from build123d import *

# Parameters (mm, degrees)
EXTRUDE_1_DEPTH     = 9
SKETCH_2_W          = 12.1
SKETCH_2_H          = 5
CUT_EXTRUDE_1_DEPTH = 0.9
SKETCH_3_R          = 29.401854515
SKETCH_3_W          = 23
SKETCH_3_H          = 15
CUT_EXTRUDE_2_DEPTH = 1
CHAMFER_1_SIZE      = 2
CUT_EXTRUDE_4_DEPTH = 7.8
SKETCH_5_W          = 12.1
SKETCH_5_H          = 1.6
CUT_EXTRUDE_5_DEPTH = 5
SKETCH_6_R          = 1
SKETCH_6_R_2        = 0.9
CUT_EXTRUDE_6_DEPTH = 3
CUT_EXTRUDE_7_DEPTH = 3
EXTRUDE_2_DEPTH     = 3
CUT_EXTRUDE_9_DEPTH = 1.7
FILLET_1_R          = 1


with BuildPart() as part:
    # Эскиз1 → Бобышка-Вытянуть1 (new body)
    with BuildSketch(Plane(origin=(0, 0, 0), x_dir=(1, 0, 0), z_dir=(0, 1, 0))):
        with BuildLine():
            Line((-13.5, 35.6), (13.5, 35.6))
            Line((13.5, 35.6), (13.5, -23.6))
            ThreePointArc((13.5, -23.6), (9.985281374, -32.085281374), (1.5, -35.6))
            Line((1.5, -35.6), (-10.5, -35.6))
            ThreePointArc((-10.5, -35.6), (-12.621320344, -34.721320344), (-13.5, -32.6))
            Line((-13.5, -32.6), (-13.5, 35.6))
        make_face()
    extrude(amount=EXTRUDE_1_DEPTH)

    # Эскиз2 → Вырез-Вытянуть1 (cut)
    with BuildSketch(Plane(origin=(0, 0, -35.6), x_dir=(-1, 0, 0), z_dir=(0, 0, -1))):
        Polygon((7.05, 6), (7.05, 0), (13.5, 0), (13.5, 9), (-13.5, 9), (-13.5, 0), (-7.05, 0), (-7.05, 6), align=None)
        with Locations((0, 2.5)):
            Rectangle(SKETCH_2_W, SKETCH_2_H)
    extrude(amount=-CUT_EXTRUDE_1_DEPTH, mode=Mode.SUBTRACT)

    # Эскиз3 → Вырез-Вытянуть2 (cut)
    with BuildSketch(Plane(origin=(0, 0, -34.7), x_dir=(-1, 0, 0), z_dir=(0, 0, -1))):
        Circle(SKETCH_3_R)
        Rectangle(SKETCH_3_W, SKETCH_3_H, mode=Mode.SUBTRACT)
    extrude(amount=-CUT_EXTRUDE_2_DEPTH, mode=Mode.SUBTRACT)

    # Фаска1
    chamfer_1_edges = [part.edges().sort_by_distance(p)[0] for p in [
        (-4.5, 9, 35.6),
        (9.985281374, 9, 32.085281374),
        (13.5, 9, -5.05),
        (-13.5, 9, -0.55),
        (-12.621320344, 9, 34.721320344),
    ]]
    chamfer(chamfer_1_edges, length=CHAMFER_1_SIZE)

    # Эскиз4 → Вырез-Вытянуть4 (cut)
    with BuildSketch(Plane.XZ):
        with BuildLine():
            Line((9.9, -33.1), (9.9, -32.1))
            Line((9.9, -32.1), (11.9, -32.1))
            Line((11.9, -32.1), (11.9, 23.6))
            ThreePointArc((11.9, 23.6), (8.853910524, 30.953910524), (1.5, 34))
            Line((1.5, 34), (-10.5, 34))
            ThreePointArc((-10.5, 34), (-11.489949494, 33.589949494), (-11.9, 32.6))
            Line((-11.9, 32.6), (-11.9, -32.1))
            Line((-11.9, -32.1), (-9.9, -32.1))
            Line((-9.9, -32.1), (-9.9, -33.1))
            Line((-9.9, -33.1), (9.9, -33.1))
        make_face()
    extrude(amount=-CUT_EXTRUDE_4_DEPTH, mode=Mode.SUBTRACT)

    # Эскиз5 → Вырез-Вытянуть5 (cut)
    with BuildSketch(Plane.XZ):
        with Locations((0, -33.9)):
            Rectangle(SKETCH_5_W, SKETCH_5_H)
    extrude(amount=-CUT_EXTRUDE_5_DEPTH, mode=Mode.SUBTRACT)

    # Эскиз6 → Вырез-Вытянуть6 (cut)
    with BuildSketch(Plane(origin=(0, 9, 0), x_dir=(1, 0, 0), z_dir=(0, 1, 0))):
        with Locations(Location((-6.5, -27.6, 0), (0, 0, 270))):
            Circle(SKETCH_6_R)
        with Locations(Location((1.5, -23.6, 0), (0, 0, 270))):
            Circle(SKETCH_6_R_2)
    extrude(amount=-CUT_EXTRUDE_6_DEPTH, mode=Mode.SUBTRACT)

    # Эскиз8 → Вырез-Вытянуть7 (cut)
    with BuildSketch(Plane(origin=(13.5, 0, 0), x_dir=(0, 0, -1), z_dir=(1, 0, 0))):
        with BuildLine():
            Line((-22.65, 2.2), (-22.65, 0))
            Line((-22.65, 0), (-18.15, 0))
            Line((-18.15, 0), (-18.15, 2.2))
            ThreePointArc((-18.15, 2.2), (-20.4, 4.45), (-22.65, 2.2))
        make_face()
    extrude(amount=-CUT_EXTRUDE_7_DEPTH, mode=Mode.SUBTRACT)

    # Эскиз10 → Бобышка-Вытянуть2 (add)
    with BuildSketch(Plane(origin=(0, 9, 0), x_dir=(1, 0, 0), z_dir=(0, 1, 0))):
        with BuildLine():
            Line((-11.5, 33.7), (11.5, 33.7))
            Line((11.5, 33.7), (4.619956712, 26.186537456))
            ThreePointArc((4.619956712, 26.186537456), (0, 24.3), (-4.619956712, 26.186537456))
            Line((-4.619956712, 26.186537456), (-11.5, 33.7))
        make_face()
    extrude(amount=-EXTRUDE_2_DEPTH)

    # Эскиз9 → Вырез-Вытянуть9 (cut)
    with BuildSketch(Plane(origin=(0, 9, 0), x_dir=(1, 0, 0), z_dir=(0, 1, 0))):
        with BuildLine():
            Line((-10, 33.7), (-3.5, 27.329208434))
            ThreePointArc((-3.5, 27.329208434), (0, 25.9), (3.5, 27.329208434))
            Line((3.5, 27.329208434), (10, 33.7))
            Line((10, 33.7), (-10, 33.7))
        make_face()
    extrude(amount=-CUT_EXTRUDE_9_DEPTH, mode=Mode.SUBTRACT)

    # Скругление1
    fillet_1_edges = [part.edges().sort_by_distance(p)[0] for p in [
        (-10, 8.25, -33.7),
        (10, 8.25, -33.7),
    ]]
    fillet(fillet_1_edges, radius=FILLET_1_R)


solid = part.part
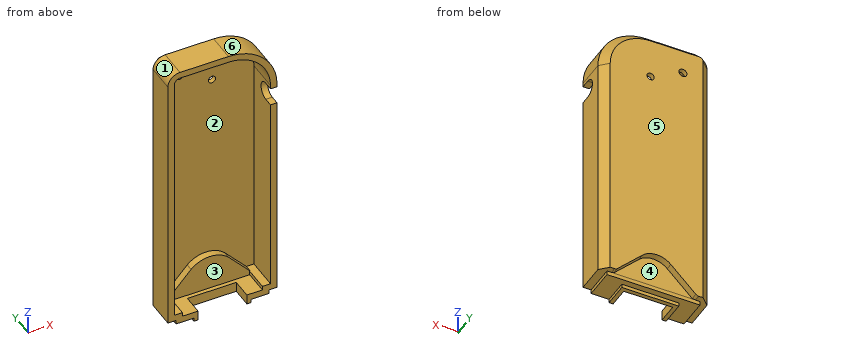
Geometry check sheet. Reference: the model listing, model coordinates, mm. Face numbers are marked on the shaded views. A direction names the side the tool comes from. Round coordinates to 2 decimals unless told otherwise and drop trailing zeros. Order: outer loops, then holes, each group sorted by start corner. A loop starts at its lowest first (then second) coordinate and runs counter-clockwise, first axis right, second up. Notation, with made-up numbers: (50.25, 19) - (62.25, 19) arc R27 ccw to (62.25, 49) - close; hole circle Ø1 at (39, 49). An arc over 180 degrees is marked (long way). One line per question, with ' | ' between items. Start each with the question number.
(1) Sectioned sample at C-C on x = -0.5. Record the cut outline in (y, z).
(2) Release check for a two-part mould opening along X. For the marked faces 3, 4, 5 and 6 record: released by +X, released by -X, zero draft, split by the parting line, or undercut.
(3) Depth check by flat-ended pin: pin 1 Ø0.9 at (x, y) = (12, 4) entering from -Z; pin 2 Ø1.2 at (y, z) = (3.5, -34.5) entering from +X; pin 3 Ø2 at (x, y) = (10.5, 4.5) entering from +Z. Enter the tip coordinate at first touch or a pass-through.
(4) Thickness scan on L1, parallel to Z at x = -7.75, y = 2.75; L2, parallel to X at y = 1, z = -19; L3, parallel to Z at x = 0.5, y = 5.25. Record the ranges inside material, lowest first. Write a range as [from, to].
(5) Access from +Z, -Z, +X, -X, +Y, -Y to the whole of each face (thin tool, end or side, straight path). Record for the marked faces 1 and 2.
(6) Sectioned sample at D-D on z = 20.4. Record the cut outline in (x, y).
(7) Sectioned sample at B-B on z = -12. Record the cut outline in (x, y).
Conclusion:
1) outline: (0, 34) - (7.8, 34) - (7.8, -24.32) - (6, -24.32) - (6, -33.1) - (5, -33.1) - (5, -35.6) - (6, -35.6) - (6, -34.7) - (7.5, -34.7) - (7.5, -33.7) - (7.3, -33.7) - (7.3, -25.93) - (9, -25.93) - (9, 33.6) - (7, 35.6) - (0, 35.6) - close
2) face 3: undercut | face 4: undercut | face 5: zero draft | face 6: released by +X
3) pin 1: stops at z = -33.7 | pin 2: stops at x = 11.5 | pin 3: stops at z = 32.54
4) L1: z = [-34.7, -33.1], [34, 35.6] | L2: x = [-13.5, -11.9], [11.9, 13.5] | L3: z = [-35.6, -33.1], [34, 35.6]
5) face 1: +Z, -X, +Y, -Y | face 2: -Y
6) outline: (-13.5, 0) - (-11.9, 0) - (-11.9, 7.8) - (11.9, 7.8) - (11.9, 4.45) - (13.5, 4.45) - (13.5, 7) - (11.5, 9) - (-11.5, 9) - (-13.5, 7) - close
7) outline: (-13.5, 0) - (-11.9, 0) - (-11.9, 7.8) - (11.9, 7.8) - (11.9, 0) - (13.5, 0) - (13.5, 7) - (11.5, 9) - (-11.5, 9) - (-13.5, 7) - close
